Could you check a few things on this model? Use its own coordinates, in mm. A direction names the side the tool comes from. Coordinates: 2 decimals unless noted, no trailing zeros. Loops run counter-clockwise (first coordinate to the right, second up) from the corner with the lowest first, then second, coordinate; pieces in that order, holes last. Notation, with made-up numbers: (15.5, 50) - (30.5, 50) arc R13 cw to (30.5, 54) - close; hole circle Ø3 at (89, 5). An arc over 180 degrees is marked (long way). Put each result on its own line as item: value. Start each with the question number.
```python
from build123d import *

# Parameters (mm, degrees)
SKETCH1_W           = 210
SKETCH1_H           = 192
BOSS_EXTRUDE1_DEPTH = 105
SKETCH2_W           = 206
SKETCH2_H           = 206
CUT_EXTRUDE1_DEPTH  = 190


with BuildPart() as part:
    # Sketch1 → Boss-Extrude1 (new body, symmetric)
    with BuildSketch(Plane.XY):
        Rectangle(SKETCH1_W, SKETCH1_H)
    extrude(amount=BOSS_EXTRUDE1_DEPTH, both=True)

    # Sketch2 → Cut-Extrude1 (cut)
    with BuildSketch(Plane(origin=(0, 96, 0), x_dir=(1, 0, 0), z_dir=(0, 1, 0))):
        Rectangle(SKETCH2_W, SKETCH2_H)
    extrude(amount=-CUT_EXTRUDE1_DEPTH, mode=Mode.SUBTRACT)


solid = part.part
```
(1) Which directions (+Z, -Z, +X, -X, +Y, -Y) give clear straight access to the entire face, cutting with the end or side of a thin tool? Please do faces 5 (the flat face through (-1, 2, 103)), 6 (the flat face through (-1, 1, -105)).
(2) I need wall thicknesses on L1, parallel to Z at x = 3, y = 20; L2, parallel to Y at x = -83, z = -72.5. Which ranges of each line are inside material? Lowest first, please. Write a range as [from, to].
(3) I want a section at A-A on y = 8.5. List the corners of the cut face in (x, z) for me, and give its area (3 significant figures).
(4) If we mould it in two halves opening along X, with no side actions, what happens to faces 1 (the flat face through (-1, -96, 1)), 2 (the flat face through (105, -1, 1)), 3 (the flat face through (103, 2, 1)), 4 (the flat face through (-103, 2, 1))? For each: pulls with the +X half, pulls with the -X half, needs draft (parallel to the pull), parting line crosses it, or undercut.
(5) For pin 1 Ø3 at (x, z) = (26.5, 51.5) entering from +Y, with a flat end and sliding along its axis, tell me the tip position at first contact or that it passes through.
(6) I want a section at C-C on z = 41.5. List the corners of the cut face in (x, y) for me.
(7) I want a section at B-B on x = 78.5. List the corners of the cut face in (y, z) for me.
Answer sheet:
1. face 5: +Y
1. face 6: -Z, +X, -X, +Y, -Y
2. L1: z = [-105, -103], [103, 105]
2. L2: y = [-96, -94]
3. outline: (-105, -105) - (105, -105) - (105, 105) - (-105, 105) - close; hole (-103, -103) - (103, -103) - (103, 103) - (-103, 103) - close
3. area: 1,660 mm^2
4. face 1: needs draft
4. face 2: pulls with the +X half
4. face 3: undercut
4. face 4: undercut
5. pin 1: stops at y = -94
6. outline: (-105, -96) - (105, -96) - (105, 96) - (103, 96) - (103, -94) - (-103, -94) - (-103, 96) - (-105, 96) - close
7. outline: (-96, -105) - (96, -105) - (96, -103) - (-94, -103) - (-94, 103) - (96, 103) - (96, 105) - (-96, 105) - close
